Source: three-view drawing plus pictorial views. Frame: mm from the lowest corner of the part. Give positions to 0.01 mm unless a question says otherwise; leave off trailing zeros. Order: outer loops, then holes, each group sorted by start corner. A loop starts at its lowest first (then second) coordinate and runs counter-clockwise, first axis right, second up.
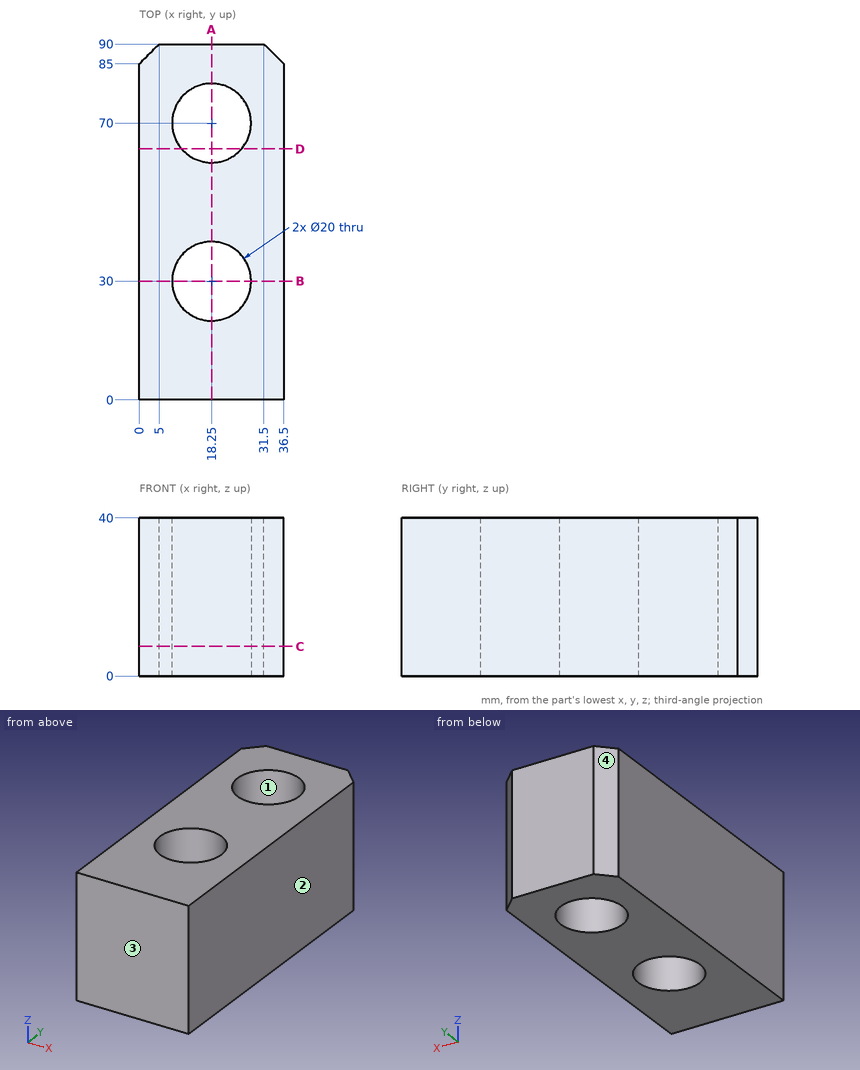
1) First-contact query: pin 1 Ø18 at (x, y) = (18.25, 70) entering from -Z; pin 2 Ø6 at (x, y) = (26.5, 48.5) entering from -Z. Flat tips, straight axial feed; report the tip coordinate or a pass-through.
Checks:
pin 1: passes through
pin 2: stops at z = 0
2) Section query A-A on x = 18.25. Output: boundary loops of the cut face in (y, z), and give its area (3 significant figures).
Checks:
outline: (0, 0) - (20, 0) - (20, 40) - (0, 40) - close; (40, 0) - (60, 0) - (60, 40) - (40, 40) - close; (80, 0) - (90, 0) - (90, 40) - (80, 40) - close
area: 2,000 mm2
3) Ray query, L1, parallel to Y at x = 18, z = 17; L2, parallel to X at y = 31, z = 31; L3, parallel to X at y = 78, z = 19.5. Return the intervals inside material, ascending.
Checks:
L1: y = 0 to 20, 40 to 60, 80 to 90
L2: x = 0 to 8.3, 28.2 to 36.5
L3: x = 0 to 12.25, 24.25 to 36.5
4) Section query D-D on y = 63.5. Output: boundary loops of the cut face in (x, z).
Checks:
outline: (0, 0) - (10.65, 0) - (10.65, 40) - (0, 40) - close; (25.85, 0) - (36.5, 0) - (36.5, 40) - (25.85, 40) - close
5) Section query C-C on z = 7.5. Output: boundary loops of the cut face in (x, y), and give its area (3 significant figures).
Checks:
outline: (0, 0) - (36.5, 0) - (36.5, 85) - (31.5, 90) - (5, 90) - (0, 85) - close; hole circle Ø20 at (18.25, 30); hole circle Ø20 at (18.25, 70)
area: 2,630 mm2
6) Pull-direction query (Y, two-part tool) for the marked faces 1, 2, 3 and 4; classes: +Y half, -Y half, draft (parallel to the pull), parting line (faces both ways), or undercut.
Checks:
face 1: undercut
face 2: draft
face 3: -Y half
face 4: +Y half
7) Section query B-B on y = 30. Output: boundary loops of the cut face in (x, z).
Checks:
outline: (0, 0) - (8.25, 0) - (8.25, 40) - (0, 40) - close; (28.25, 0) - (36.5, 0) - (36.5, 40) - (28.25, 40) - close
